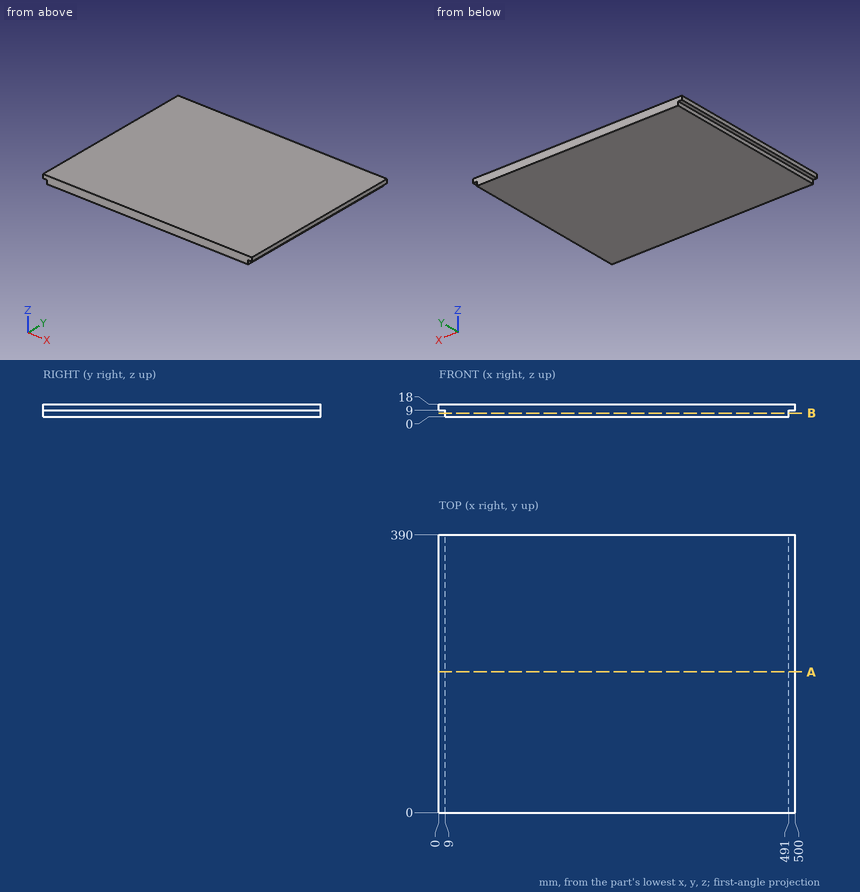
Part print with two shaded views. Sizes in mm from the minimum x, y, z corner. Round coordinates to 2 decimals unless told otherwise and drop trailing zeros. Order: outer loops, then holes, each group sorted by start corner. A loop starts at its lowest first (then second) coordinate and runs counter-clockwise, first axis right, second up. Notation, with made-up numbers: M -17,81 L 11,81 A27 ccw 11,113 Z; hole C 17,85 d7. An arc over 180 degrees is marked long. Put each result on its own line as item: value. Start each with the question number.
1. Slice it at A-A on y = 197.5. List the corners of the cut face in (x, z), then the cut area to 3 significant figures.
2. Slice it at B-B on z = 5.25. List the corners of the cut face in (x, y).
3. Drill centre line: probe 1 along X at (y, z) = (355, 4.75). Where is it in solid material? Low to high. Write a range as [from, to].
4. Drop flat-ended pins along their axis: pin 1 (2.5 mm diameter, centred on y = 240.5, z = 6.5, fed in from +X); pin 2 (4.5 mm diameter, centred on x = 494, y = 287, fed in from -Z); pin 3 (1.5 mm diameter, centred on y = 164, z = 4.5, fed in from -X). Give the stop position or say it passes through.
Findings:
1. outline: M 0,9 L 9,9 L 9,0 L 491,0 L 491,9 L 500,9 L 500,18 L 0,18 Z
1. area: 8,840 mm2
2. outline: M 9,0 L 491,0 L 491,390 L 9,390 Z
3. probe 1: [9, 491]
4. pin 1: x = 491
4. pin 2: z = 9
4. pin 3: x = 9
